from build123d import *

# Parameters (mm, degrees)
F1_DEPTH = 2.6
F2_R     = 1.5
F3_R     = 1


with BuildPart() as f1:
    # F0 (on Top) → F1 (new body)
    with BuildSketch(Plane.XY):
        with BuildLine():
            ThreePointArc((-6, 28.25), (-6.512563, 29.487437), (-7.75, 30))
            ThreePointArc((-7.75, 30), (-8.987437, 27.012563), (-6, 28.25))
        make_face()
        Polygon((-7.75, 33.5), (-13.5, 33.5), (-13.5, 5.3), (-15.5, 5.3), (-15.5, 0), (0, 0), (0, 5.3), (-2, 5.3), (-2, 33.5), align=None)
        with BuildLine():
            Line((-6.15, 12.9), (-6.15, 9.6))
            ThreePointArc((-6.15, 9.6), (-7.75, 8), (-9.35, 9.6))
            Line((-9.35, 9.6), (-9.35, 12.9))
            ThreePointArc((-9.35, 12.9), (-7.75, 14.5), (-6.15, 12.9))
        make_face(mode=Mode.SUBTRACT)
        with BuildLine():
            ThreePointArc((-6, 28.25), (-8.987437, 27.012563), (-7.75, 30))
            ThreePointArc((-7.75, 30), (-6.512563, 29.487437), (-6, 28.25))
        make_face(mode=Mode.SUBTRACT)
    extrude(amount=F1_DEPTH)

    # F2
    f2_edges = [f1.edges().sort_by_distance(p)[0] for p in [
        (-13.5, 33.5, 1.3),
        (-2, 33.5, 1.3),
    ]]
    fillet(f2_edges, radius=F2_R)

    # F3
    f3_edges = [f1.edges().sort_by_distance(p)[0] for p in [
        (0, 0, 1.3),
        (-15.5, 0, 1.3),
    ]]
    fillet(f3_edges, radius=F3_R)


solid = f1.part
Verification items for the finished model (mm, model axes). A direction names the side the tool comes from. Round coordinates to 2 decimals unless told otherwise and drop trailing zeros. Loops run counter-clockwise (first coordinate to the right, second up) from the corner with the lowest first, then second, coordinate; pieces in that order, holes last. Notation, with made-up numbers: (-36, 60.25) - (22, 60.25) arc R12 cw to (22, 77.25) - close; hole circle Ø3 at (18, 77.5). An arc over 180 degrees is marked (long way). Use a Markdown table: item, result. Add a question column.
1. Section check B-B, the plane y = 22. Record the boundary of the cut face in (x, z).
2. Section check A-A, the plane z = 0.3. Record the boundary of the cut face in (x, y).
3. Gauge pin test, flat ends, axial feed: pin 1 (1.5 mm diameter, centred on y = 19, z = 1, fed in from +X); pin 2 (1 mm diameter, centred on x = -15, z = 0.5, fed in from +Y); pin 3 (0.8 mm diameter, centred on y = 13.5, z = 1, fed in from -X). Record the tip position at first contact, or that the pin passes through.
4. Thickness scan on probe 1 along Y at (x, z) = (-7.75, 0.65); probe 2 along X at (y, z) = (28.25, 1.05); probe 3 along X at (y, z) = (10, 1.7). Record the ranges inside material, lowest first. Write a range as [from, to].
5. Access from +Z, -Z, +X, -X, +Y, -Y to the whole of each face (thin tool, end or side, straight path). Record for faces 5 (the face through (-14, 5.3, 1)), 6 (the face through (-6.15, 11, 1)), 7 (the face through (-1, 5.3, 1)).
6. Release check for a two-part mould opening along X. For faces 1 (the face through (-9.35, 11, 1)), 2 (the face through (-2, 18, 1)), 3 (the face through (-8, 17, 2.6)), 4 (the face through (-15.5, 3, 1)) record: released by +X, released by -X, zero draft, split by the parting line, or undercut.
Checks:
| question | item | result |
|---|---|---|
| 1 | outline | (-13.5, 0) - (-2, 0) - (-2, 2.6) - (-13.5, 2.6) - close |
| 2 | outline | (-15.5, 1) arc R1 ccw to (-14.5, 0) - (-1, 0) arc R1 ccw to (0, 1) - (0, 5.3) - (-2, 5.3) - (-2, 32) arc R1.5 ccw to (-3.5, 33.5) - (-12, 33.5) arc R1.5 ccw to (-13.5, 32) - (-13.5, 5.3) - (-15.5, 5.3) - close; hole circle Ø3.5 at (-7.75, 28.25); hole (-9.35, 9.6) arc R1.6 ccw to (-6.15, 9.6) - (-6.15, 12.9) arc R1.6 ccw to (-9.35, 12.9) - close |
| 3 | pin 1 | stops at x = -2 |
| 3 | pin 2 | stops at y = 5.3 |
| 3 | pin 3 | stops at x = -13.5 |
| 4 | probe 1 | y = [0, 8], [14.5, 26.5], [30, 33.5] |
| 4 | probe 2 | x = [-13.5, -9.5], [-6, -2] |
| 4 | probe 3 | x = [-13.5, -9.35], [-6.15, -2] |
| 5 | face 5 | +Z, -Z, -X, +Y |
| 5 | face 6 | +Z, -Z |
| 5 | face 7 | +Z, -Z, +X, +Y |
| 6 | face 1 | undercut |
| 6 | face 2 | released by +X |
| 6 | face 3 | zero draft |
| 6 | face 4 | released by -X |
